CAD build for the part. Positions are in the model's coordinates, mm. A direction names the side the tool comes from. Round coordinates to 2 decimals unless told otherwise and drop trailing zeros. Order: outer loops, then holes, each group sorted by start corner. A loop starts at its lowest first (then second) coordinate and runs counter-clockwise, first axis right, second up. Notation, with made-up numbers: (10, 17.25) - (23, 17.25) arc R23 ccw to (23, 29.25) - close; hole circle Ø9 at (50.25, 56.5). An arc over 180 degrees is marked (long way). Write item = value, one per line.
from build123d import *

# Parameters (mm, degrees)
BOSS_EXTRUDE1_DEPTH      = 20
BOSS_EXTRUDE1_DEPTH_BACK = 20
SKETCH1_R                = 5
BOSS_EXTRUDE2_DEPTH      = 20
BOSS_EXTRUDE2_DEPTH_BACK = 20
SKETCH2_R                = 5


with BuildPart() as part:
    # Sketch1 → Boss-Extrude1 (new, two sides: drawn at the far end of the back side and taken through both)
    with BuildSketch(Plane(origin=(0, 0, 0), x_dir=(0, 0, -1), z_dir=(1, 0, 0)).offset(-BOSS_EXTRUDE1_DEPTH_BACK)):
        Circle(SKETCH1_R)
    extrude(amount=BOSS_EXTRUDE1_DEPTH + BOSS_EXTRUDE1_DEPTH_BACK)

    # Sketch2 → Boss-Extrude2 (add, two sides: drawn at the far end of the back side and taken through both)
    with BuildSketch(Plane(origin=(0, 0, 0), x_dir=(1, 0, 0), z_dir=(0, 1, 0)).offset(-BOSS_EXTRUDE2_DEPTH_BACK)):
        with Locations(Location((0, 0, 0), (0, 0, 270))):
            Circle(SKETCH2_R)
    extrude(amount=BOSS_EXTRUDE2_DEPTH + BOSS_EXTRUDE2_DEPTH_BACK)


solid = part.part
(1) Band-saw the part on D-D on y = 3.5. List the corners of the cut face in (x, z), plus the area to 3 significant figures.
Solved:
outline = (-20, -3.57) - (-3.5, -3.57) arc R5 ccw to (3.5, -3.57) - (20, -3.57) - (20, 3.57) - (3.5, 3.57) arc R5 ccw to (-3.5, 3.57) - (-20, 3.57) - close
area = 299 mm²
(2) Drop flat-ended pins along their axis: pin 1 (1 mm diameter, centred on x = 7, y = -4.5, fed in from +Z); pin 2 (1.5 mm diameter, centred on x = -4.5, y = -4.5, fed in from -Z); pin 3 (5 mm diameter, centred on x = -6.5, y = 10.5, fed in from -Z). Give the stop position or say it passes through.
Solved:
pin_1 = 3
pin_2 = -3.31
pin_3 = -3
(3) Probe line 1 along Y through (x, z) = (15, -0.25); line 2 along Z through (x, y) = (2.5, -15). List the from-to ranges inside material, lowest first.
Solved:
line_1 = -4.99 to 4.99
line_2 = -4.33 to 4.33
(4) Band-saw the part on A-A on y = -3. List the corners of the cut face in (x, z), plus the area to 3 significant figures.
Solved:
outline = (-20, -4) - (-3, -4) arc R5 ccw to (3, -4) - (20, -4) - (20, 4) - (3, 4) arc R5 ccw to (-3, 4) - (-20, 4) - close
area = 328 mm²
(5) Band-saw the part on B-B on z = 0. List the corners of the cut face in (x, y), plus the area to 3 significant figures.
Solved:
outline = (-20, -5) - (-5, -5) - (-5, -20) - (5, -20) - (5, -5) - (20, -5) - (20, 5) - (5, 5) - (5, 20) - (-5, 20) - (-5, 5) - (-20, 5) - close
area = 700 mm²
(6) Band-saw the part on C-C on x = -9.5. List the corners of the cut face in (y, z), plus the area to 3 significant figures.
Solved:
outline = circle Ø10 at (0, 0)
area = 78.5 mm²
(7) Tool access for faces 1 (the cylindrical face through (-12, 0, 5)), 2 (the cylindrical face through (0, -12, -5)), 3 (the cylindrical face through (-3, 12, -4)), 4 (the cylindrical face through (12, -3, 4)): list every direction of +Z, -Z, +X, -X, +Y, -Y with a clear straight run to the whole face (end or side of a thin tool).
Solved:
face_1 = -X
face_2 = -Y
face_3 = +Y
face_4 = +X
